Build history of the part. All positions in model axes, mm. A direction names the side the tool comes from. Round coordinates to 2 decimals unless told otherwise and drop trailing zeros. Write each loop counter-clockwise with the first axis right and the second up, starting at its lowest first coordinate (ties: lowest second). Pieces come first, ordered by that corner, then holes. Notation, with made-up numbers: (-25, 70) - (30, 70) arc R16 cw to (30, 92) - close; hole circle Ø6 at (12.25, 46). An arc over 180 degrees is marked (long way). One line per question, with ' | ' between items.
from build123d import *

# Parameters (mm, degrees)
SKETCH1_R           = 21
SKETCH1_R_2         = 20
BOSS_EXTRUDE1_DEPTH = 3.5
SKETCH2_R           = 3.55
SKETCH2_R_2         = 6.55
SKETCH2_R_3         = 8.5
SKETCH2_W           = 11.2
SKETCH2_H           = 4.84
BOSS_EXTRUDE2_DEPTH = 3


with BuildPart() as part:
    # Sketch1 → Boss-Extrude1 (new body)
    with BuildSketch(Plane(origin=(0, 0, 0), x_dir=(1, 0, 0), z_dir=(0, 1, 0))):
        Circle(SKETCH1_R)
        Circle(SKETCH1_R_2, mode=Mode.SUBTRACT)
    extrude(amount=BOSS_EXTRUDE1_DEPTH)

    # Sketch2 → Boss-Extrude2 (add)
    with BuildSketch(Plane(origin=(0, 3.5, 0), x_dir=(1, 0, 0), z_dir=(0, 1, 0))):
        Polygon((-37, 37), (-37, -37), (37, -37), (37, 37), (24.5, 37), (24.5, 59), (-24.5, 59), (-24.5, 37), align=None)
        with Locations((-23.55, -23.55)):
            Circle(SKETCH2_R, mode=Mode.SUBTRACT)
        Circle(SKETCH2_R_2, mode=Mode.SUBTRACT)
        with Locations((23.55, -23.55)):
            Circle(SKETCH2_R, mode=Mode.SUBTRACT)
        with Locations((-23.55, 23.55)):
            Circle(SKETCH2_R, mode=Mode.SUBTRACT)
        with Locations((23.55, 23.55)):
            Circle(SKETCH2_R, mode=Mode.SUBTRACT)
        with Locations((13.76, 47)):
            Circle(SKETCH2_R_3, mode=Mode.SUBTRACT)
        with Locations((-13.76, 47)):
            Circle(SKETCH2_R_3, mode=Mode.SUBTRACT)
        with Locations((0, 52.78)):
            Rectangle(SKETCH2_W, SKETCH2_H, mode=Mode.SUBTRACT)
    extrude(amount=BOSS_EXTRUDE2_DEPTH)


solid = part.part
Q1. Pull direction Z, two halves, no side cores. Call faces 1 (the flat face through (24.5, 5, -48)), 2 (the cylindrical face through (-0.853, 4.979, -6.494)), 3 (the flat face through (-31, 5, -37)): +Z half, -Z half, draft (parallel to the pull), parting line (faces both ways), or undercut.
Found:
face 1: draft | face 2: undercut | face 3: -Z half
Q2. Saw through at C-C, the plane y = 5.25. State how many separate pieces and enclosed holes the cut face has, then the cut area to 3 significant figures.
Found:
separate pieces: 1 | enclosed holes: 8 | area: 5,750 mm^2
Q3. Drill centre lines: L1, parallel to Z at x = 23.55, y = 5.4; L2, parallel to Z at x = 0, y = 0.95; L3, parallel to X at y = 5.2, z = -23.55. Where is each one in solid material? Low to high. Write a range as from..to.
Found:
L1: -59..-27.1, -20..20, 27.1..37 | L2: -21..-20, 20..21 | L3: -37..-27.1, -20..20, 27.1..37
Q4. Drop flat-ended pins along their axis: pin 1 (9 mm diameter, centred on x = -23.55, z = 23.55, fed in from -Y); pin 2 (3.5 mm diameter, centred on y = 4.5, z = -52.5, fed in from -X); pin 3 (3.5 mm diameter, centred on x = 28.5, y = 5.5, fed in from -Z); pin 4 (13.5 mm diameter, centred on x = -13.76, z = -47, fed in from -Y). Give the stop position or say it passes through.
Found:
pin 1: y = 3.5 | pin 2: x = -24.5 | pin 3: z = -37 | pin 4: through
Q5. Saw through at A-A, the plane z = -23.55. List the corners of the cut face in (x, y).
Found:
outline: (-37, 3.5) - (-27.1, 3.5) - (-27.1, 6.5) - (-37, 6.5) - close; (-20, 3.5) - (20, 3.5) - (20, 6.5) - (-20, 6.5) - close; (27.1, 3.5) - (37, 3.5) - (37, 6.5) - (27.1, 6.5) - close
Q6. Saw through at D-D, the plane z = 0. List the corners of the cut face in (x, y).
Found:
outline: (-37, 3.5) - (-21, 3.5) - (-21, 0) - (-20, 0) - (-20, 3.5) - (-6.55, 3.5) - (-6.55, 6.5) - (-37, 6.5) - close; (6.55, 3.5) - (20, 3.5) - (20, 0) - (21, 0) - (21, 3.5) - (37, 3.5) - (37, 6.5) - (6.55, 6.5) - close
Q7. Which spindle directions (+Z, -Z, +X, -X, +Y, -Y) get a long thin tool onto all of the face, cutting with end or side? Do faces 4 (the flat face through (-5, 3.5, -5)), 5 (the flat face through (-1, 6.5, -12)), 6 (the flat face through (31, 5, -37)), 7 (the flat face through (0, 5, -50.36)). Say none if no direction does.
Found:
face 4: -Y | face 5: +Z, -Z, +X, -X, +Y | face 6: -Z, +X, +Y, -Y | face 7: +Y, -Y
Q8. Saw through at B-B, the plane x = 0. List the corners of the cut face in (y, z).
Found:
outline: (0, -21) - (3.5, -21) - (3.5, -50.36) - (6.5, -50.36) - (6.5, -6.55) - (3.5, -6.55) - (3.5, -20) - (0, -20) - close; (0, 20) - (3.5, 20) - (3.5, 6.55) - (6.5, 6.55) - (6.5, 37) - (3.5, 37) - (3.5, 21) - (0, 21) - close; (3.5, -59) - (6.5, -59) - (6.5, -55.2) - (3.5, -55.2) - close
